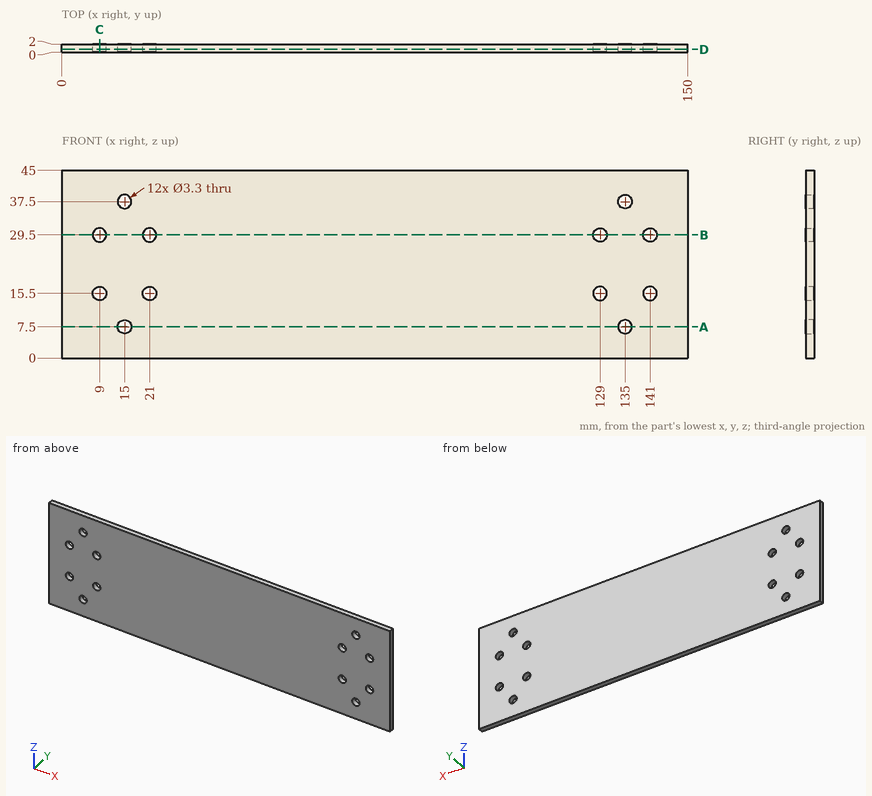
For this review, use the dimensioned drawing (mm, ordinates from the lowest corner) and the shaded views. Coordinates: 2 decimals unless noted, no trailing zeros. Order: outer loops, then holes, each group sorted by start corner. A loop starts at its lowest first (then second) coordinate and runs counter-clockwise, first axis right, second up. Notation, with made-up numbers: M -36,24 L -25,24 A31 ccw -25,61 Z; hole C 60,44.25 d8. An arc over 180 degrees is marked long. Answer as a JSON object with one key per item and string values. Group by question number.
1) Wall thickness on L1, parallel to Z at x = 141, y = 0.95; L2, parallel to X at y = 1.45, z = 15.5; L3, parallel to X at y = 1.15, z = 7.5: over which ranges is each line inside the solid? List them lowest first.
2) Add section D-D, the plane y = 0.7. Count the separate pieces of the cut face and the enclosed holes in it, then the cut area to 3 significant figures.
3) For pin 1 (2 mm diameter, centred on x = 135, z = 7.5, fed in from -Y), flat-tipped, find the tip position at first contact; note if it passes through.
4) Add section B-B, the plane z = 29.5. Write out the cut boundary in (x, y), then the cut area to 3 significant figures.
5) Add section C-C, the plane x = 9. Write out the cut boundary in (y, z), then the cut area to 3 significant figures.
6) Add section A-A, the plane z = 7.5. Write out the cut boundary in (x, y), then the cut area to 3 significant figures.
Computed values:
{
 "1": {"L1": "z = 0 to 13.85, 17.15 to 27.85, 31.15 to 45", "L2": "x = 0 to 7.35, 10.65 to 19.35, 22.65 to 127.35, 130.65 to 139.35, 142.65 to 150", "L3": "x = 0 to 13.35, 16.65 to 133.35, 136.65 to 150"},
 "2": {"separate pieces": "1", "enclosed holes": "12", "area": "6,650 mm^2"},
 "3": {"pin 1": "passes through"},
 "4": {"outline": "M 0,0 L 7.35,0 L 7.35,2 L 0,2 Z; M 10.65,0 L 19.35,0 L 19.35,2 L 10.65,2 Z; M 22.65,0 L 127.35,0 L 127.35,2 L 22.65,2 Z; M 130.65,0 L 139.35,0 L 139.35,2 L 130.65,2 Z; M 142.65,0 L 150,0 L 150,2 L 142.65,2 Z", "area": "274 mm^2"},
 "5": {"outline": "M 0,0 L 2,0 L 2,13.85 L 0,13.85 Z; M 0,17.15 L 2,17.15 L 2,27.85 L 0,27.85 Z; M 0,31.15 L 2,31.15 L 2,45 L 0,45 Z", "area": "76.8 mm^2"},
 "6": {"outline": "M 0,0 L 13.35,0 L 13.35,2 L 0,2 Z; M 16.65,0 L 133.35,0 L 133.35,2 L 16.65,2 Z; M 136.65,0 L 150,0 L 150,2 L 136.65,2 Z", "area": "287 mm^2"}
}
